```python
from build123d import *

# Parameters (mm, degrees)
F0_W         = 50
F0_H         = 38
F0_W_2       = 10
F0_H_2       = 5
F0_W_3       = 16.5
F0_H_3       = 16.5
F1_DEPTH     = 25
F2_R         = 3
F3_DEPTH     = 7.4141664952
F4_R         = 3
F5_DEPTH     = 7.571767807
F6_R         = 15
F7_T1_DEPTH  = 35.5
F7_T3_DEPTH  = 20
F7_T6_ANGLE  = 90
F7_T8_ANGLE  = 90
F7_T10_ANGLE = 90
F7_T12_ANGLE = 90


# Not quite as in the source:
# - a fillet or chamfer that OpenCascade refuses, or shapes differently, is made with other operations: its cross-section is extruded or revolved along the edge and cut away or added


with BuildPart() as f1:
    # F0 (on Front) → F1 (new body)
    with BuildSketch(Plane.XZ):
        Rectangle(F0_W, F0_H)
        with Locations((-17.2914686799, -13.928232193)):
            Rectangle(F0_W_2, F0_H_2, mode=Mode.SUBTRACT)
        with Locations((17.7085313201, -13.928232193)):
            Rectangle(F0_W_2, F0_H_2, mode=Mode.SUBTRACT)
        Rectangle(F0_W_3, F0_H_3, mode=Mode.SUBTRACT)
        with Locations((0, 14.0858335048)):
            Rectangle(F0_W_2, F0_H_2, mode=Mode.SUBTRACT)
    extrude(amount=F1_DEPTH)

    # F2 (on face) → F3 (cut, through all)
    with BuildSketch(Plane.XY.offset(19)):
        with Locations((0, -12.5)):
            Circle(F2_R)
    extrude(amount=-F3_DEPTH, mode=Mode.SUBTRACT)

    # F4 (on face) → F5 (cut, through all)
    with BuildSketch(Plane(origin=(0, 0, -19), x_dir=(1, 0, 0), z_dir=(0, 0, -1))):
        with Locations((-17.2914686799, 11)):
            Circle(F4_R)
        with Locations((17.7085313201, 11)):
            Circle(F4_R)
    extrude(amount=-F5_DEPTH, mode=Mode.SUBTRACT)

    # F6
    f6_edges = [f1.edges().sort_by_distance(p)[0] for p in [
        (-25, -12.5, 19),
        (25, -12.5, 19),
    ]]
    fillet(f6_edges, radius=F6_R)

    # F7: fillet of radius 5 on 10 edges, made by hand

    # F7_s2 → F7_t1 (cut)
    with BuildSketch(Plane.XY.offset(-31.5)):
        with BuildLine():
            ThreePointArc((-20, 0), (-23.5355339059, -1.4644660941), (-25, -5))
            Line((-25, -5), (-25, 0))
            Line((-25, 0), (-20, 0))
        make_face()
        with BuildLine():
            ThreePointArc((20, 0), (23.5355339059, -1.4644660941), (25, -5))
            Line((25, -5), (25, 0))
            Line((25, 0), (20, 0))
        make_face()
        with BuildLine():
            ThreePointArc((20, -25), (23.5355339059, -23.5355339059), (25, -20))
            Line((25, -20), (25, -25))
            Line((25, -25), (20, -25))
        make_face()
        with BuildLine():
            ThreePointArc((-20, -25), (-23.5355339059, -23.5355339059), (-25, -20))
            Line((-25, -20), (-25, -25))
            Line((-25, -25), (-20, -25))
        make_face()
    extrude(amount=F7_T1_DEPTH, mode=Mode.SUBTRACT)

    # F7_s4 → F7_t3 (cut)
    with BuildSketch(Plane.YZ.offset(-10)):
        with BuildLine():
            ThreePointArc((-20, 19), (-23.5355339059, 17.5355339059), (-25, 14))
            Line((-25, 14), (-25, 19))
            Line((-25, 19), (-20, 19))
        make_face()
        with BuildLine():
            ThreePointArc((-5, 19), (-1.4644660941, 17.5355339059), (0, 14))
            Line((0, 14), (0, 19))
            Line((0, 19), (-5, 19))
        make_face()
    extrude(amount=F7_T3_DEPTH, mode=Mode.SUBTRACT)

    # F7_s5 → F7_t6 (revolve, cut)
    with BuildSketch(Plane.YZ.offset(-10)):
        with BuildLine():
            ThreePointArc((0, 14), (-1.4644660941, 17.5355339059), (-5, 19))
            Line((-5, 19), (0, 19))
            Line((0, 19), (0, 14))
        make_face()
    revolve(axis=Axis((-10, 0, 4), (0, -1, 0)), revolution_arc=F7_T6_ANGLE, mode=Mode.SUBTRACT)

    # F7_s7 → F7_t8 (revolve, cut)
    with BuildSketch(Plane.YZ.offset(10)):
        with BuildLine():
            ThreePointArc((0, 14), (-1.4644660941, 17.5355339059), (-5, 19))
            Line((-5, 19), (0, 19))
            Line((0, 19), (0, 14))
        make_face()
    revolve(axis=Axis((10, 0, 4), (0, 1, 0)), revolution_arc=F7_T8_ANGLE, mode=Mode.SUBTRACT)

    # F7_s9 → F7_t10 (revolve, cut)
    with BuildSketch(Plane.YZ.offset(10)):
        with BuildLine():
            ThreePointArc((-20, 19), (-23.5355339059, 17.5355339059), (-25, 14))
            Line((-25, 14), (-25, 19))
            Line((-25, 19), (-20, 19))
        make_face()
    revolve(axis=Axis((10, -25, 4), (0, 1, 0)), revolution_arc=F7_T10_ANGLE, mode=Mode.SUBTRACT)

    # F7_s11 → F7_t12 (revolve, cut)
    with BuildSketch(Plane.YZ.offset(-10)):
        with BuildLine():
            ThreePointArc((-20, 19), (-23.5355339059, 17.5355339059), (-25, 14))
            Line((-25, 14), (-25, 19))
            Line((-25, 19), (-20, 19))
        make_face()
    revolve(axis=Axis((-10, -25, 4), (0, -1, 0)), revolution_arc=F7_T12_ANGLE, mode=Mode.SUBTRACT)


solid = f1.part
```
The listing builds one solid part. Answer for the finished solid, in the listing's coordinates (mm). A direction names the side the tool comes from. Coordinates: 2 decimals unless noted, no trailing zeros. Write each loop counter-clockwise with the first axis right and the second up, starting at its lowest first coordinate (ties: lowest second). Pieces come first, ordered by that corner, then holes. Notation, with made-up numbers: (78.5, 1) - (97.5, 1) arc R12 cw to (97.5, 18) - close; hole circle Ø5 at (70, 53.25). An arc over 180 degrees is marked (long way). One line per item, written item: value.
1) A tool of negligible diameter and unlimited length cuts with its end or side. For faces 4 (the flat face through (0, -9, 19)), 5 (the flat face through (-3.4, -12.3, 16.586)), 6 (the cylindrical face through (-14.5, -9.9, -17.7)), from which of +Z, -Z, +X, -X, +Y, -Y can it reach the whole face along a straight path? Write none if from no direction.
Geometry check:
face 4: +Z, +X, -X, +Y, -Y
face 5: +Y, -Y
face 6: -Z
2) Find section A-A (x = 0). Give the vertices of the cut face in (y, z), and give its area (3 significant figures).
Geometry check:
outline: (-25, -19) - (0, -19) - (0, -8.25) - (-25, -8.25) - close; (-25, 8.25) - (0, 8.25) - (0, 11.59) - (-25, 11.59) - close; (-24.28, 16.59) - (-15.5, 16.59) - (-15.5, 19) - (-20, 19) arc R5 ccw to start; (-9.5, 16.59) - (-0.72, 16.59) arc R5 ccw to (-5, 19) - (-9.5, 19) - close
area: 388 mm2
3) Find section C-C (z = -10.5). Give the vertices of the cut face in (x, y), and give its area (3 significant figures).
Geometry check:
outline: (-25, -20) arc R5 ccw to (-20, -25) - (20, -25) arc R5 ccw to (25, -20) - (25, -5) arc R5 ccw to (20, 0) - (-20, 0) arc R5 ccw to (-25, -5) - close
area: 1,230 mm2
4) Each of these flat-tipped pins is pushed along its axis until it touches: pin 1 Ø5.5 at (y, z) = (-8, 13.5) entering from -X; pin 2 Ø12 at (y, z) = (-10.5, 15) entering from +X; pin 3 Ø7 at (x, y) = (-17.29, -11) entering from +Z; pin 4 Ø5 at (x, z) = (4, -2) entering from +Y. Where does it stop, or does it pass through?
Geometry check:
pin 1: stops at x = -23.4
pin 2: stops at x = 24.14
pin 3: stops at z = 18.51
pin 4: passes through
5) Consider line 1 along X through (y, z) = (-11, -17.2); line 2 along Z through (x, y) = (2, -6.25); line 3 along X through (y, z) = (-2.75, -14). Determine where each line is inside the solid, lowest interval first. Write a range as from..to.
Geometry check:
line 1: x = -25..-20.29, -14.29..14.71, 20.71..25
line 2: z = -19..-8.25, 8.25..11.59, 16.59..19
line 3: x = -24.47..-22.29, -12.29..12.71, 22.71..24.47
6) Find section B-B (y = -16.25). Give the vertices of the cut face in (x, z).
Geometry check:
outline: (-25, -19) - (25, -19) - (25, 4) arc R15 ccw to (10, 19) - (-10, 19) arc R15 ccw to (-25, 4) - close; hole (-22.29, -16.43) - (-12.29, -16.43) - (-12.29, -11.43) - (-22.29, -11.43) - close; hole (-8.25, -8.25) - (8.25, -8.25) - (8.25, 8.25) - (-8.25, 8.25) - close; hole (-5, 11.59) - (5, 11.59) - (5, 16.59) - (-5, 16.59) - close; hole (12.71, -16.43) - (22.71, -16.43) - (22.71, -11.43) - (12.71, -11.43) - close
7) For a pull along Z with two mould halves and no side action, classify faces 1 (the flat face through (22.709, -12, -14)), 2 (the cylindrical face through (20.5, -9.9, -17.7)), 3 (the cylindrical face through (-20.72, -12.6, 14.49)) as pulls with the +Z half, pulls with the -Z half, needs draft (parallel to the pull), parting line crosses it, or undercut.
Geometry check:
face 1: undercut
face 2: needs draft
face 3: pulls with the +Z half
